Part model, mm, in its own coordinate system. Give positions to 0.01 mm unless a question says otherwise; leave off trailing zeros. Order: outer loops, then holes, each group sorted by start corner. A loop starts at its lowest first (then second) coordinate and runs counter-clockwise, first axis right, second up. Notation, with made-up numbers: M 41.25,66.5 L 91.25,66.5 A14 cw 91.25,92.5 Z; hole C 43.5,-3.75 d2. An arc over 180 degrees is marked long. Answer as a JSON object with one key per item and string values.
from build123d import *

# Parameters (mm, degrees)
SKETCH1_W                = 40
SKETCH1_H                = 40
SKETCH1_W_2              = 34
SKETCH1_H_2              = 34
EXTRUDE_THIN1_DEPTH      = 1200
FILLET1_R                = 0.5
FILLET2_R                = 3
F_8_0_8_DIAMETER_HOLE1_D = 8
F_8_0_8_DIAMETER_HOLE2_D = 8


with BuildPart() as part:
    # Sketch1 → Extrude-Thin1 (new body)
    with BuildSketch(Plane.XY):
        Rectangle(SKETCH1_W, SKETCH1_H)
        Rectangle(SKETCH1_W_2, SKETCH1_H_2, mode=Mode.SUBTRACT)
    extrude(amount=EXTRUDE_THIN1_DEPTH)

    # Fillet1
    fillet1_edges = [part.edges().sort_by_distance(p)[0] for p in [
        (17, -17, 600),
        (17, 17, 600),
        (-17, 17, 600),
        (-17, -17, 600),
    ]]
    fillet(fillet1_edges, radius=FILLET1_R)

    # Fillet2
    fillet2_edges = [part.edges().sort_by_distance(p)[0] for p in [
        (20, -20, 600),
        (-20, -20, 600),
        (-20, 20, 600),
        (20, 20, 600),
    ]]
    fillet(fillet2_edges, radius=FILLET2_R)

    # Ø8.0 (8) Diameter Hole1 (through all)
    with Locations(Plane(origin=(0, 20, 0), x_dir=(1, 0, 0), z_dir=(0, 1, 0))):
        with Locations((0, -20), (0, -1180)):
            Hole(F_8_0_8_DIAMETER_HOLE1_D / 2)

    # Ø8.0 (8) Diameter Hole2 (through all)
    with Locations(Plane(origin=(0, 20, 0), x_dir=(1, 0, 0), z_dir=(0, 1, 0))):
        with Locations((-8, -1060), (-8, -140)):
            Hole(F_8_0_8_DIAMETER_HOLE2_D / 2)


solid = part.part
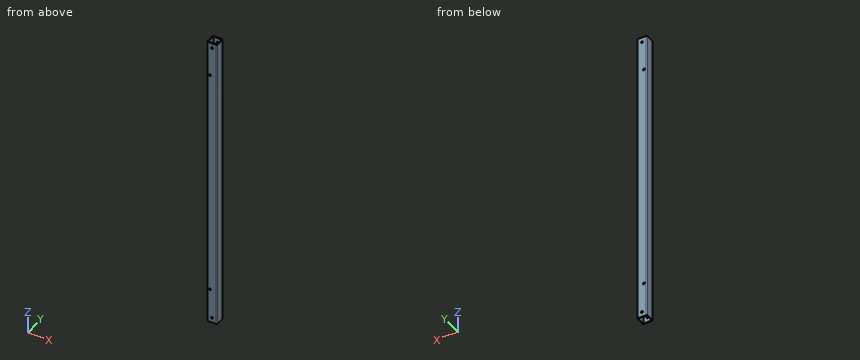
1. Cut at A-A on y = -1.5. Give the cut face in (x, z).
Worked answers:
{"outline": "M -20,0 L -17,0 L -17,1200 L -20,1200 Z; M 17,0 L 20,0 L 20,1200 L 17,1200 Z"}
2. Pin check, flat tip, straight feed: P1, Ø1, axis at x = 15.5, y = 14, coming from the -Z side. Stop position of the tip, or through.
Worked answers:
{"P1": "passes through"}
3. Probe line 1 along Z through (x, y) = (-8, -18.3); line 2 along Y through (x, z) = (-13, 635.5). List the from-to ranges inside material, lowest first.
Worked answers:
{"line 1": "z = 0 to 136, 144 to 1056, 1064 to 1200", "line 2": "y = -20 to -17, 17 to 20"}
4. Cut at B-B on z = 1125. Give the cut face in (x, y).
Worked answers:
{"outline": "M -20,-17 A3 ccw -17,-20 L 17,-20 A3 ccw 20,-17 L 20,17 A3 ccw 17,20 L -17,20 A3 ccw -20,17 Z; hole M -17,-16.5 A0.5 ccw -16.5,-17 L 16.5,-17 A0.5 ccw 17,-16.5 L 17,16.5 A0.5 ccw 16.5,17 L -16.5,17 A0.5 ccw -17,16.5 Z"}
